from build123d import *

# Parameters (mm, degrees)
BOSS_EXTRUDE1_DEPTH     = 6.35
SKETCH2_R               = 6.35
BOSS_EXTRUDE2_DEPTH     = 101.6
SKETCH3_R               = 12.7
SKETCH3_R_2             = 6.35
CUT_EXTRUDE1_DEPTH      = 101.6
SKETCH4_R               = 12.7
CUT_EXTRUDE2_DEPTH      = 7.35
SKETCH5_R               = 12.7
CUT_EXTRUDE3_DEPTH      = 7.35
CUT_EXTRUDE3_DEPTH_BACK = 7.35


with BuildPart() as part:
    # Sketch1 → Boss-Extrude1 (new body)
    with BuildSketch(Plane(origin=(0, 0, 0), x_dir=(1, 0, 0), z_dir=(0, 1, 0))):
        Polygon((-76.2, 76.2), (-76.2, -76.2), (76.2, -76.2), (76.2, -25.4), (-25.4, 76.2), align=None)
    extrude(amount=BOSS_EXTRUDE1_DEPTH)

    # Sketch2 → Boss-Extrude2 (add)
    with BuildSketch(Plane.ZY.offset(76.2)):
        with Locations((0, 6.35)):
            Circle(SKETCH2_R)
    extrude(amount=BOSS_EXTRUDE2_DEPTH)

    # Sketch3 → Cut-Extrude1 (cut)
    with BuildSketch(Plane(origin=(0, 6.35, 0), x_dir=(1, 0, 0), z_dir=(0, 1, 0))):
        with Locations((-50.8, -38.1)):
            Circle(SKETCH3_R)
        with Locations((50.8, -50.8)):
            Circle(SKETCH3_R_2)
    extrude(amount=-CUT_EXTRUDE1_DEPTH, mode=Mode.SUBTRACT)

    # Sketch4 → Cut-Extrude2 (cut, through all)
    with BuildSketch(Plane(origin=(0, 6.35, 0), x_dir=(1, 0, 0), z_dir=(0, 1, 0))):
        with Locations((-53.956209782, 0)):
            Circle(SKETCH4_R)
    extrude(amount=-CUT_EXTRUDE2_DEPTH, mode=Mode.SUBTRACT)

    # Sketch5 → Cut-Extrude3 (cut, two sides)
    with BuildSketch(Plane(origin=(0, 6.35, 0), x_dir=(1, 0, 0), z_dir=(0, 1, 0))) as cut_extrude3_sk:
        with Locations((-53.956209782, 50.8)):
            Circle(SKETCH5_R)
    extrude(amount=CUT_EXTRUDE3_DEPTH, mode=Mode.SUBTRACT)
    extrude(cut_extrude3_sk.sketch, amount=-CUT_EXTRUDE3_DEPTH_BACK, mode=Mode.SUBTRACT)


solid = part.part
Can you work these out from the model? Positions are in its coordinate system, mm. A direction names the side the tool comes from. Coordinates: 2 decimals unless noted, no trailing zeros. Write each loop counter-clockwise with the first axis right and the second up, starting at its lowest first coordinate (ties: lowest second). Pieces come first, ordered by that corner, then holes.
Q1. For P1, Ø11.5, axis at x = 50.8, z = 50.8, coming from the +Y side; P2, Ø7, axis at y = 10, z = -2, coming from the +X side; P3, Ø7, axis at y = 3, z = -55.5, coming from the -X side; P4, Ø3, axis at x = -127, y = 3.5, coming from the -Z side, each with a flat end and sliding along its axis, tell me the tip position at first contact or that it passes through.
Results found:
P1: passes through
P2: stops at x = -76.2
P3: stops at x = -76.2
P4: stops at z = -6.2
Q2. Which directions (+Z, -Z, +X, -X, +Y, -Y) give clear straight access to the entire face, cutting with the end or side of a thin tool? Please do faces 4 (the face through (-126.289, 12.646, -0.827)), 5 (the face through (-38.686, 3.219, 34.285)), 6 (the face through (-76.2, 9, 0)).
Results found:
face 4: -X
face 5: +Y, -Y
face 6: +Z, -Z, +X, +Y
Q3. Please list where these lines run through material, in increasing order: L1, parallel to Z at x = -50.8, y = 1.75; L2, parallel to X at y = 2.75, z = 0; L3, parallel to Z at x = 50.8, y = 3.
Results found:
L1: z = -76.2 to -63.1, -38.5 to -12.3, 12.3 to 25.4, 50.8 to 76.2
L2: x = -177.8 to -66.66, -41.26 to 50.8
L3: z = 0 to 44.45, 57.15 to 76.2
Q4. Imagine slicing it at C-C, the plane x = -49.5. List the corners of the cut face in (y, z) for me, plus the area to 3 significant figures.
Results found:
outline: (0, -76.2) - (6.35, -76.2) - (6.35, -62.69) - (0, -62.69) - close; (0, -38.91) - (6.35, -38.91) - (6.35, -11.89) - (0, -11.89) - close; (0, 11.89) - (6.35, 11.89) - (6.35, 25.47) - (0, 25.47) - close; (0, 50.73) - (6.35, 50.73) - (6.35, 76.2) - (0, 76.2) - close
area: 505 mm2
Q5. If we mould it in two halves opening along Z, with no side actions, what happens to faces 1 (the face through (26.1, 3.1, -24.7)), 2 (the face through (-1, 3, 76.2)), 3 (the face through (56.857, 3.219, 48.893))? For each: +Z half, -Z half, draft (parallel to the pull), parting line (faces both ways), or undercut.
Results found:
face 1: -Z half
face 2: +Z half
face 3: undercut
Q6. Imagine slicing it at D-D, the plane x = -159.5. List the corners of the cut face in (y, z) for me.
Results found:
outline: circle Ø12.7 at (6.35, 0)
Q7. Imagine slicing it at B-B, the plane z = -53.5. List the corners of the cut face in (x, y) for me.
Results found:
outline: (-76.2, 0) - (-66.37, 0) - (-66.37, 6.35) - (-76.2, 6.35) - close; (-41.55, 0) - (-2.7, 0) - (-2.7, 6.35) - (-41.55, 6.35) - close
Q8. Imagine slicing it at A-A, the plane x = 50.8. List the corners of the cut face in (y, z) for me, plus the area to 3 significant figures.
Results found:
outline: (0, 0) - (6.35, 0) - (6.35, 44.45) - (0, 44.45) - close; (0, 57.15) - (6.35, 57.15) - (6.35, 76.2) - (0, 76.2) - close
area: 403 mm2
